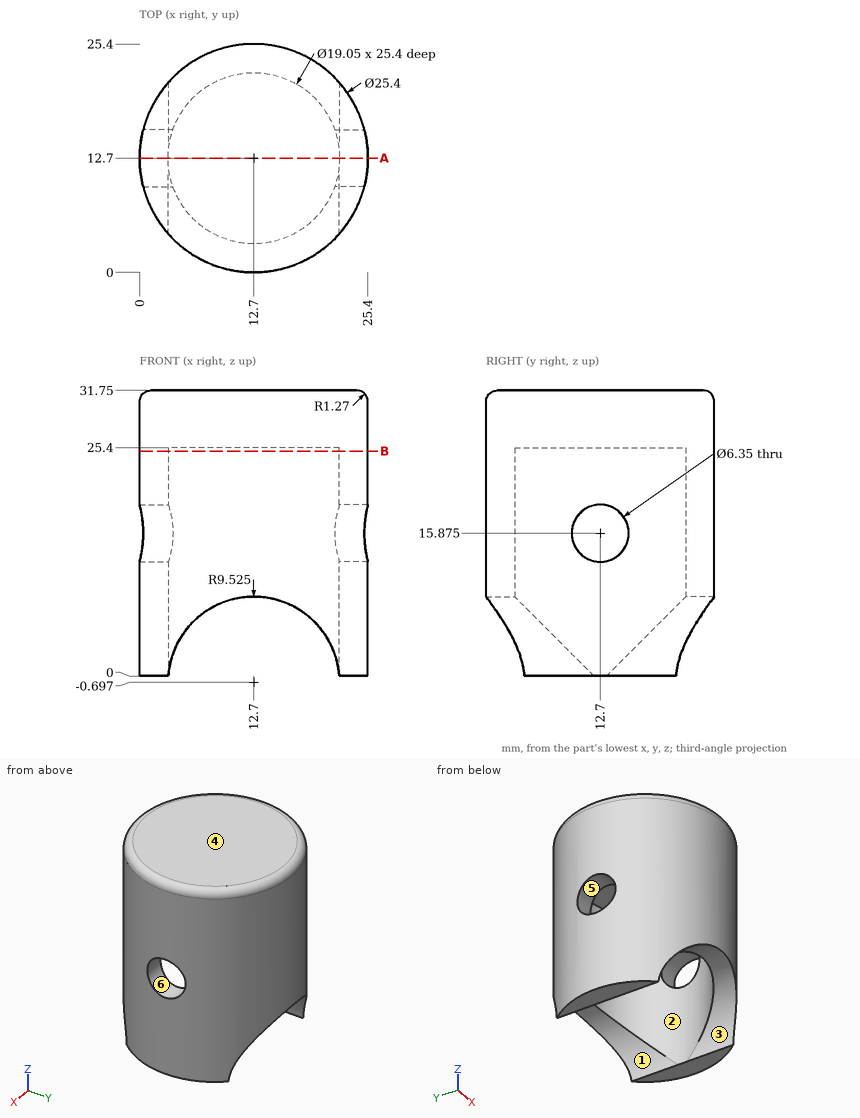
Study the drawing (mm; zero at the part's minimum x, y, z) and answer. A direction names the side the tool comes from. Round coordinates to 2 decimals unless told otherwise and drop trailing zeros. Write each loop counter-clockwise with the first axis right and the second up, starting at its lowest first coordinate (ties: lowest second). Pieces come first, ordered by that corner, then holes.
1) A tool of negligible diameter and unlimited length cuts with its end or side. For the marked faces 1 and 2, from which of +Z, -Z, +X, -X, +Y, -Y can it reach the whole face along a straight path? Write none if from no direction.
2) Given pin 1 Ø4 at (y, z) = (12.7, 15.875) entering from -X; pin 2 Ø1 at (x, y) = (4, 22) entering from -Z; pin 3 Ø1 at (x, z) = (3, 15.5) entering from +Y (3 decimals); pin 4 Ø3 at (x, z) = (23, 8.5) entering from -Y, each flat-ended and moving along its own axis, determine where each tip first touches the part or whether it passes through.
3) Straight lines are drawn through the part: line 1 (Y direction, x = 12.7, z = 13.5) (3 decimals); line 2 (Z direction, x = 11, y = 19); line 3 (X direction, y = 17, z = 20). For each, find the intervals that lie inside material, in ascending order.
4) A cutting plane is placed at A-A (y = 12.7). Give the number of separate pieces and of enclosed holes in the cut face, plus the area to 3 significant figures.
5) The mould has two halves that part along Z. Classify the marked faces 3, 4, 5 and 6: pulls with the +Z half, pulls with the -Z half, needs draft (parallel to the pull), parting line crosses it, or undercut.
6) A cutting plane is placed at B-B (z = 25). Give the vertices of the cut face in (x, y) (3 decimals), plus the area to 3 significant figures.
Completed:
1. face 1: -Z, +Y, -Y
1. face 2: -Z
2. pin 1: passes through
2. pin 2: stops at z = 2.32
2. pin 3: stops at y = 21.455
2. pin 4: stops at y = 3.54
3. line 1: y = 0 to 3.175, 22.225 to 25.4
3. line 2: z = 25.4 to 31.75
3. line 3: x = 0.75 to 4.2, 21.2 to 24.65
4. separate pieces: 3
4. enclosed holes: 0
4. area: 282 mm2
5. face 3: pulls with the -Z half
5. face 4: pulls with the +Z half
5. face 5: undercut
5. face 6: undercut
6. outline: circle Ø25.4 at (12.7, 12.7); hole circle Ø19.05 at (12.7, 12.7)
6. area: 222 mm2
